The model under review builds one solid part; all positions refer to its coordinate system, in mm. Coordinates: 2 decimals unless noted, no trailing zeros. Order: outer loops, then holes, each group sorted by start corner. A loop starts at its lowest first (then second) coordinate and runs counter-clockwise, first axis right, second up.
```python
from build123d import *

# Parameters (mm, degrees)
F1_DEPTH    = 17.78
F2_T1_DEPTH = 417.7319430625


# Not quite as in the source:
# - a fillet or chamfer that OpenCascade refuses, or shapes differently, is made with other operations: its cross-section is extruded or revolved along the edge and cut away or added


with BuildPart() as f1:
    # F0 (on Front) → F1 (new body)
    with BuildSketch(Plane.XZ):
        with BuildLine():
            Line((-162.0961189375, -1.346105228), (-162.0961189375, -39.446105228))
            Line((-162.0961189375, -39.446105228), (3.0038810625, -39.446105228))
            Line((3.0038810625, -39.446105228), (93.3108132751, 7.1072834172))
            Line((93.3108132751, 7.1072834172), (67.9108132751, 7.1072834172))
            Line((67.9108132751, 7.1072834172), (3.0038810625, -1.346105228))
            Line((3.0038810625, -1.346105228), (-43.6204448342, 0))
            add(Edge.make_bspline(
                [(-88.0704448342, -1.346105228), (-85.1866431635, -6.6508062653), (-78.8098016913, -15.013308036), (-66.0558603131, -19.2294666036), (-50.4728148138, -12.3489722112), (-48.5910698771, -6.9073382765), (-43.6204448342, 0)],
                knots=[0, 0, 0, 0, 0.2654455487, 0.4966311992, 0.7427406625, 1, 1, 1, 1], degree=3))
            Line((-88.0704448342, -1.346105228), (-162.0961189375, -1.346105228))
        make_face()
    extrude(amount=F1_DEPTH)

    # F2: fillet of radius 103.0193211336 on 1 edges, made by hand

    # F2_s2 → F2_t1 (cut)
    with BuildSketch(Plane.XZ.offset(-199.9759715313)):
        with BuildLine():
            ThreePointArc((-82.105730325, -1.346105228), (-126.4060471139, -11.3575640099), (-162.0961189375, -39.446105228))
            Line((-162.0961189375, -39.446105228), (-162.0961189375, -1.346105228))
            Line((-162.0961189375, -1.346105228), (-82.105730325, -1.346105228))
        make_face()
    extrude(amount=F2_T1_DEPTH, mode=Mode.SUBTRACT)


solid = f1.part
```
(1) We need section B-B, the plane z = -30.5. Write out the cut boundary in (x, y).
A:
outline: (-153.92, -17.78) - (20.36, -17.78) - (20.36, 0) - (-153.92, 0) - close
(2) For pin 1 Ø3 at (y, z) = (-5, -13) entering from -X; pin 2 Ø5 at (x, y) = (26.5, -14.5) entering from +Z; pin 3 Ø1.5 at (y, z) = (-7.5, -15.5) entering from +X, all flat-tipped, find the tip position at first contact; note any pin that passes through.
A:
pin 1: stops at x = -132.48
pin 2: stops at z = 2.04
pin 3: stops at x = 50.91
(3) Wall thickness on probe 1 along X at (y, z) = (-13.5, -14); probe 2 along Z at (x, y) = (31, -9.5); probe 3 along Z at (x, y) = (48, -4.25): over which ranges is each line inside the solid? List them lowest first.
A:
probe 1: x = -131.57 to -77.76, -55.37 to 52.37
probe 2: z = -25.01 to 2.3
probe 3: z = -16.25 to 4.51
(4) We need section A-A, the plane x = -21. Write out the cut boundary in (y, z).
A:
outline: (-17.78, -39.45) - (0, -39.45) - (0, -0.65) - (-17.78, -0.65) - close
